Geometry: final body of the model. Coordinates: model frame, mm. Coordinates: 2 decimals unless noted, no trailing zeros. Write each loop counter-clockwise with the first axis right and the second up, starting at its lowest first coordinate (ties: lowest second). Pieces come first, ordered by that corner, then holes.
Autodesk Inventor part; units mm, degrees
ref_plane "YZ Plane" through (0, 0, 0) normal (1, 0, 0) x (0, 1, 0)
ref_plane "XZ Plane" through (0, 0, 0) normal (0, 1, 0) x (-1, 0, 0)
ref_plane "XY Plane" through (0, 0, 0) normal (0, 0, 1) x (1, 0, 0)
sketch "スケッチ1" plane through (0, 0, 0) normal (0, 0, 1) x (1, 0, 0)
  line L0 (-2.8, 2.8) -> (2.8, 2.8) construction
  line L1 (2.8, 2.8) -> (2.8, -2.8) construction
  line L2 (2.8, -2.8) -> (-2.8, -2.8) construction
  line L3 (-2.8, -2.8) -> (-2.8, 2.8) construction
  circle A0 centre (-2.8, 2.8) radius 1.5
  circle A1 centre (2.8, 2.8) radius 1.5
  circle A2 centre (2.8, -2.8) radius 1.5
  circle A3 centre (-2.8, -2.8) radius 1.5
  circle A4 centre (0, 0) radius 1.3
  circle A5 centre (0, 0) radius 6
  dimension "d0" = 3
  dimension "d1" = 3
  dimension "d2" = 3
  dimension "d3" = 3
  dimension "d4" = 5.6
  dimension "d5" = 2.6
  dimension "d6" = 12
extrude "押し出し1" add sketch "スケッチ1" along normal blind 8
properties part number "脚最終段カム1" material "アルミニウム 7075"
Item 1: Section D-D, the plane z = 5.25. Output: boundary loops of the cut face in (x, y), plus the area to 3 significant figures.
Derived:
outline: circle Ø12 at (0, 0); hole circle Ø3 at (-2.8, -2.8); hole circle Ø3 at (-2.8, 2.8); hole circle Ø2.6 at (0, 0); hole circle Ø3 at (2.8, -2.8); hole circle Ø3 at (2.8, 2.8)
area: 79.5 mm2
Item 2: Pin query (flat end, axial travel): pin 1 (1.5 mm diameter, centred on x = -3.5, z = 4.5, fed in from +Y); pin 2 (4 mm diameter, centred on x = 4, z = 2, fed in from +Y). Return the tip coordinate at first contact, or that it passes through.
Derived:
pin 1: stops at y = 5.33
pin 2: stops at y = 5.66
Item 3: Material intervals for probe 1 along Y at (x, z) = (-2.8, 3); probe 2 along X at (y, z) = (2.25, 5.5); probe 3 along X at (y, z) = (2.75, 1.25), sorted ascending.
Derived:
probe 1: y = -5.31 to -4.3, -1.3 to 1.3, 4.3 to 5.31
probe 2: x = -5.56 to -4.2, -1.4 to 1.4, 4.2 to 5.56
probe 3: x = -5.33 to -4.3, -1.3 to 1.3, 4.3 to 5.33
Item 4: Pull-direction query (Y, two-part tool) for faces 1 (the cylindrical face through (-6, 0, 4)), 2 (the cylindrical face through (1.6, -1.9, 3.9)), 3 (the flat face through (1.2, -1.2, 8)); classes: released by +Y, released by -Y, zero draft, split by the parting line, or undercut.
Derived:
face 1: split by the parting line
face 2: undercut
face 3: zero draft
Item 5: Section C-C, the plane x = 1.75. Output: boundary loops of the cut face in (y, z).
Derived:
outline: (-5.74, 0) - (-3.87, 0) - (-3.87, 8) - (-5.74, 8) - close; (-1.73, 0) - (1.73, 0) - (1.73, 8) - (-1.73, 8) - close; (3.87, 0) - (5.74, 0) - (5.74, 8) - (3.87, 8) - close
Item 6: Section A-A, the plane y = 0. Output: boundary loops of the cut face in (x, z), plus the area to 3 significant figures.
Derived:
outline: (-6, 0) - (-1.3, 0) - (-1.3, 8) - (-6, 8) - close; (1.3, 0) - (6, 0) - (6, 8) - (1.3, 8) - close
area: 75.2 mm2
